Check sheet for the modelled part. Datum: model origin and axes. Units: mm. A direction names the side the tool comes from. Coordinates: 2 decimals unless noted, no trailing zeros. Write each loop counter-clockwise with the first axis right and the second up, starting at its lowest first coordinate (ties: lowest second). Pieces come first, ordered by that corner, then holes. Notation, with made-up numbers: M -26.75,50.25 L -10.75,50.25 A16 ccw -10.75,62.25 Z; hole C -21.5,-6.5 d7. An arc over 180 degrees is marked long. Answer as CSV lines item,"result". Start each with the question number.
Q1. Mould release check, pull along Y, two halves, no side actions. Record for faces 1 (the flat face through (13, 5, 2.9)), 2 (the flat face through (-10, 5, 2.9)), 3 (the flat face through (-19.837, 4, 19)), 4 (the flat face through (-21.941, -5.069, 28.925)): pulls with the +Y half, pulls with the -Y half, needs draft (parallel to the pull), parting line crosses it, or undercut.
Q2. Access from +Z, -Z, +X, -X, +Y, -Y to the whole of each face (thin tool, end or side, straight path). Record for faces 5 (the flat face through (-10, 16.296, 26)), 6 (the flat face through (-11.035, -12.121, 4.472)).
Q3. Sectioned sample at B-B, the plane z = 29.25. Record the cut outline in (x, y).
Q4. Sectioned sample at D-D, the plane z = 8. Record the cut outline in (x, y), then the cut area to 3 significant figures.
Q5. Sectioned sample at C-C, the plane y = 1. Record the cut outline in (x, z), then the cut area to 3 significant figures.
Q6. Depth check by flat-ended pin: pin 1 Ø8 at (x, y) = (14.5, 7) entering from +Z; pin 2 Ø13 at (x, z) = (7, 27) entering from -Y; pin 3 Ø2 at (x, z) = (17.54, 44.75) entering from +Y. Enter the tip coordinate at first touch or a pass-through.
Q7. Thickness scan on line 1 along X through (y, z) = (15, 29); line 2 along X through (y, z) = (0.5, 12.5); line 3 along Y through (x, z) = (11, 12.5). Record the ranges inside material, lowest first. Write a range as from..to.
Q8. Sectioned sample at A-A, the plane z = 44.75. Record the cut outline in (x, y), then the cut area to 3 significant figures.
from build123d import *

# Parameters (mm, degrees)
F0_W      = 52
F0_H      = 40
F1_DEPTH  = 6
F2_W      = 52
F2_H      = 2.2
F3_DEPTH  = 46.5
F5_DEPTH  = 4.1
F7_DEPTH  = 4.15
F8_R      = 11.75
F8_R_2    = 1.85
F9_DEPTH  = 25
F10_R     = 2.5
F11_DEPTH = 25
F13_DEPTH = 3.1


with BuildPart() as f1:
    # F0 (on Top) → F1 (new body)
    with BuildSketch(Plane.XY):
        with Locations((2.012877, -3.704458)):
            Rectangle(F0_W, F0_H)
    extrude(amount=F1_DEPTH)

    # F2 (on face) → F3 (join)
    with BuildSketch(Plane.XY.offset(6)):
        with Locations((2.012877, 15.195542)):
            Rectangle(F2_W, F2_H)
    extrude(amount=F3_DEPTH)

    # F4 (on face) → F5 (join)
    with BuildSketch(Plane.YZ.offset(28.012877)):
        Polygon((14.095542, 52.5), (-23.704458, 6), (14.095542, 6), align=None)
    extrude(amount=-F5_DEPTH)

    # F6 (on face) → F7 (join)
    with BuildSketch(Plane(origin=(-23.987123, 0, 0), x_dir=(0, -1, 0), z_dir=(-1, 0, 0))):
        Polygon((23.704458, 6), (-14.095542, 52.5), (-14.095542, 6), align=None)
    extrude(amount=-F7_DEPTH)

    # F8 (on face) → F9 (cut)
    with BuildSketch(Plane.XZ.offset(-14.095542)):
        with Locations((2.037877, 29.25)):
            Circle(F8_R)
        with Locations((17.537877, 44.75)):
            Circle(F8_R_2)
        with Locations((-13.462123, 44.75)):
            Circle(F8_R_2)
        with Locations((-13.462123, 13.75)):
            Circle(F8_R_2)
        with Locations((17.537877, 13.75)):
            Circle(F8_R_2)
    extrude(amount=-F9_DEPTH, mode=Mode.SUBTRACT)

    # F10 (on face) → F11 (cut)
    with BuildSketch(Plane(origin=(0, 0, 0), x_dir=(1, 0, 0), z_dir=(0, 0, -1))):
        with Locations((13.512877, 15.204458)):
            Circle(F10_R)
        with Locations((-9.487123, 15.204458)):
            Circle(F10_R)
        with Locations((-9.487123, -7.795542)):
            Circle(F10_R)
        with Locations((13.512877, -7.795542)):
            Circle(F10_R)
    extrude(amount=-F11_DEPTH, mode=Mode.SUBTRACT)

    # F12 (on face) → F13 (cut)
    with BuildSketch(Plane.XY.offset(6)):
        Polygon((13.312949, -11.225761), (9.96726, -13.388251), (10.167187, -17.366948), (13.712804, -19.183154), (17.058493, -17.020664), (16.858566, -13.041967), align=None)
        Polygon((13.712804, 11.774239), (10.167187, 9.958033), (9.96726, 5.979336), (13.312949, 3.816846), (16.858566, 5.633052), (17.058493, 9.611749), align=None)
        Polygon((-13.03274, -17.020664), (-9.687051, -19.183154), (-6.141434, -17.366948), (-5.941507, -13.388251), (-9.287196, -11.225761), (-12.832813, -13.041967), align=None)
        Polygon((-5.941507, 5.979336), (-6.141434, 9.958033), (-9.687051, 11.774239), (-13.03274, 9.611749), (-12.832813, 5.633052), (-9.287196, 3.816846), align=None)
    extrude(amount=-F13_DEPTH, mode=Mode.SUBTRACT)


solid = f1.part
Output:
1,face 1,"undercut"
1,face 2,"undercut"
1,face 3,"needs draft"
1,face 4,"pulls with the -Y half"
2,face 5,"+Z, -Z, +X, -X, +Y"
2,face 6,"+Z"
3,outline,"M -23.99,-4.8 L -19.84,-4.8 L -19.84,14.1 L -9.71,14.1 L -9.71,16.3 L -23.99,16.3 Z; M 13.79,14.1 L 23.91,14.1 L 23.91,-4.8 L 28.01,-4.8 L 28.01,16.3 L 13.79,16.3 Z"
4,outline,"M -23.99,-22.08 L -19.84,-22.08 L -19.84,14.1 L 23.91,14.1 L 23.91,-22.08 L 28.01,-22.08 L 28.01,16.3 L -23.99,16.3 Z"
4,area,"413 mm^2"
5,outline,"M -23.99,0 L 28.01,0 L 28.01,36.39 L 23.91,36.39 L 23.91,6 L -19.84,6 L -19.84,36.39 L -23.99,36.39 Z"
5,area,"563 mm^2"
6,pin 1,"stops at z = 6"
6,pin 2,"stops at y = 14.1"
6,pin 3,"passes through"
7,line 1,"x = -23.99..-9.71, 13.79..28.01"
7,line 2,"x = -23.99..-19.84, 23.91..28.01"
7,line 3,"y = 14.1..16.3"
8,outline,"M -23.99,7.8 L -19.84,7.8 L -19.84,14.1 L -15.31,14.1 L -15.31,16.3 L -23.99,16.3 Z; M -11.61,14.1 L 15.69,14.1 L 15.69,16.3 L -11.61,16.3 Z; M 19.39,14.1 L 23.91,14.1 L 23.91,7.8 L 28.01,7.8 L 28.01,16.3 L 19.39,16.3 Z"
8,area,"150 mm^2"
